The figure shows three views and two pictorial views of one solid part (mm, origin at its lowest corner). Answer the questions. Coordinates: 2 decimals unless noted, no trailing zeros. Loops run counter-clockwise (first coordinate to the right, second up) from the corner with the lowest first, then second, coordinate; pieces in that order, holes last. Notation, with made-up numbers: M 4,-18 L 63,-18 A29 ccw 63,18 Z; hole C 62.25,-23.75 d9. An arc over 180 degrees is marked long. One line per item, written item: value. Start each with the question number.
1. The part is cut by section B-B (x = 60). Write down the section's boundary in (y, z), then the cut area to 3 significant figures.
2. The part is cut by section A-A (z = 60). Write down the section's boundary in (x, y).
3. Determine the mould class of the marked faces 1 and 2 for opening direction Y: +Y half, -Y half, draft (parallel to the pull), parting line (faces both ways), or undercut.
4. The part is cut by section C-C (y = 1.75). Write down the section's boundary in (x, z).
5. Consider probe 1 along X at (y, z) = (0.85, 105) (1 decimal); probe 2 along X at (y, z) = (0.9, 60); probe 3 along Z at (x, y) = (79, 0.85). Determine where each line is inside the solid, lowest interval first.
6. The part is cut by section D-D (z = 15). Write down the section's boundary in (x, y).
7. Flat-ended cylindrical pins translate along their axes: pin 1 (6 mm diameter, centred on x = 91.62, z = 15, fed in from +Y); pin 2 (1 mm diameter, centred on y = 2.5, z = 96, fed in from -X); pin 3 (3 mm diameter, centred on x = 28.38, z = 105, fed in from -Y); pin 4 (1.5 mm diameter, centred on y = 1.5, z = 70.5, fed in from +X). Find the tip coordinate at first contact, or state that the pin passes through.
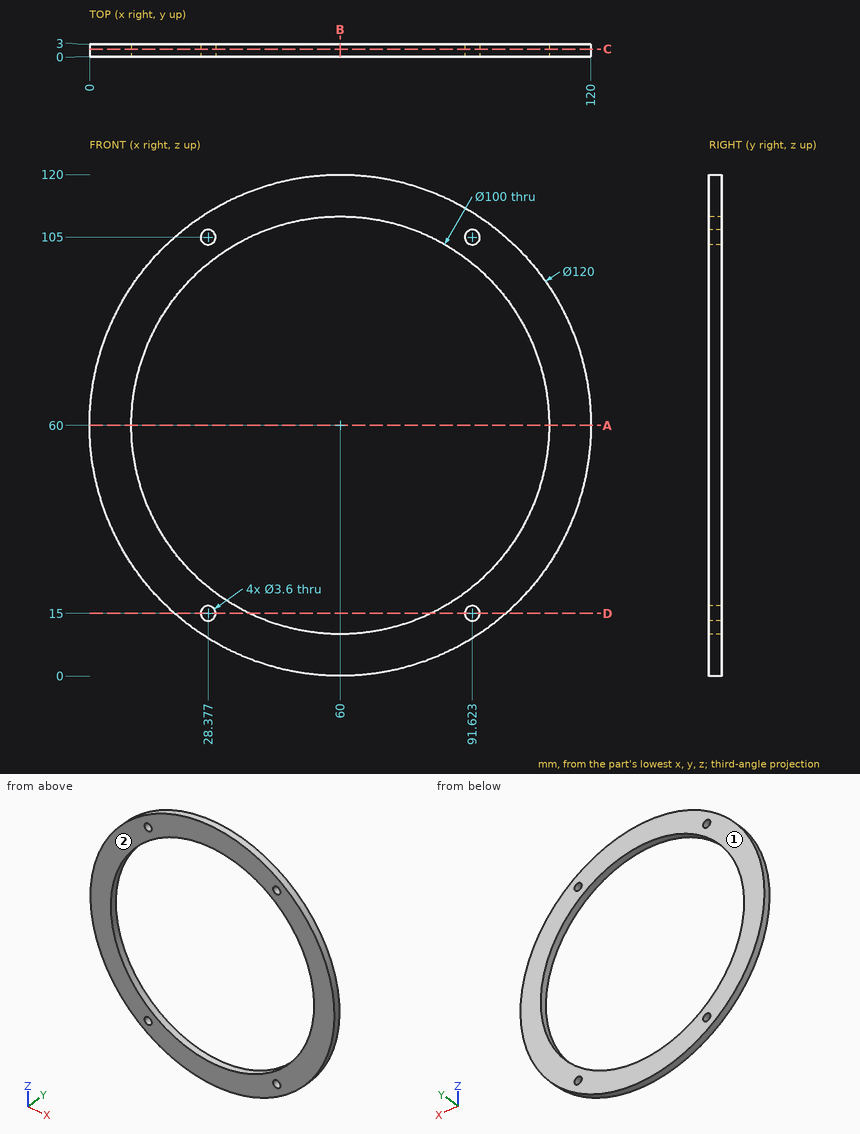
Answer block:
1. outline: M 0,0 L 3,0 L 3,10 L 0,10 Z; M 0,110 L 3,110 L 3,120 L 0,120 Z
1. area: 60.0 mm2
2. outline: M 0,0 L 10,0 L 10,3 L 0,3 Z; M 110,0 L 120,0 L 120,3 L 110,3 Z
3. face 1: +Y half
3. face 2: -Y half
4. outline: C 60,60 d120; hole C 60,60 d100; hole C 28.38,15 d3.6; hole C 28.38,105 d3.6; hole C 91.62,15 d3.6; hole C 91.62,105 d3.6
5. probe 1: x = 20.3 to 26.6, 30.2 to 38.2, 81.8 to 89.8, 93.4 to 99.7
5. probe 2: x = 0 to 10, 110 to 120
5. probe 3: z = 3.09 to 13.75, 106.25 to 116.91
6. outline: M 20.31,0 L 26.58,0 L 26.58,3 L 20.31,3 Z; M 30.18,0 L 38.21,0 L 38.21,3 L 30.18,3 Z; M 81.79,0 L 89.82,0 L 89.82,3 L 81.79,3 Z; M 93.42,0 L 99.69,0 L 99.69,3 L 93.42,3 Z
7. pin 1: stops at y = 3
7. pin 2: stops at x = 11.63
7. pin 3: passes through
7. pin 4: stops at x = 119.2
